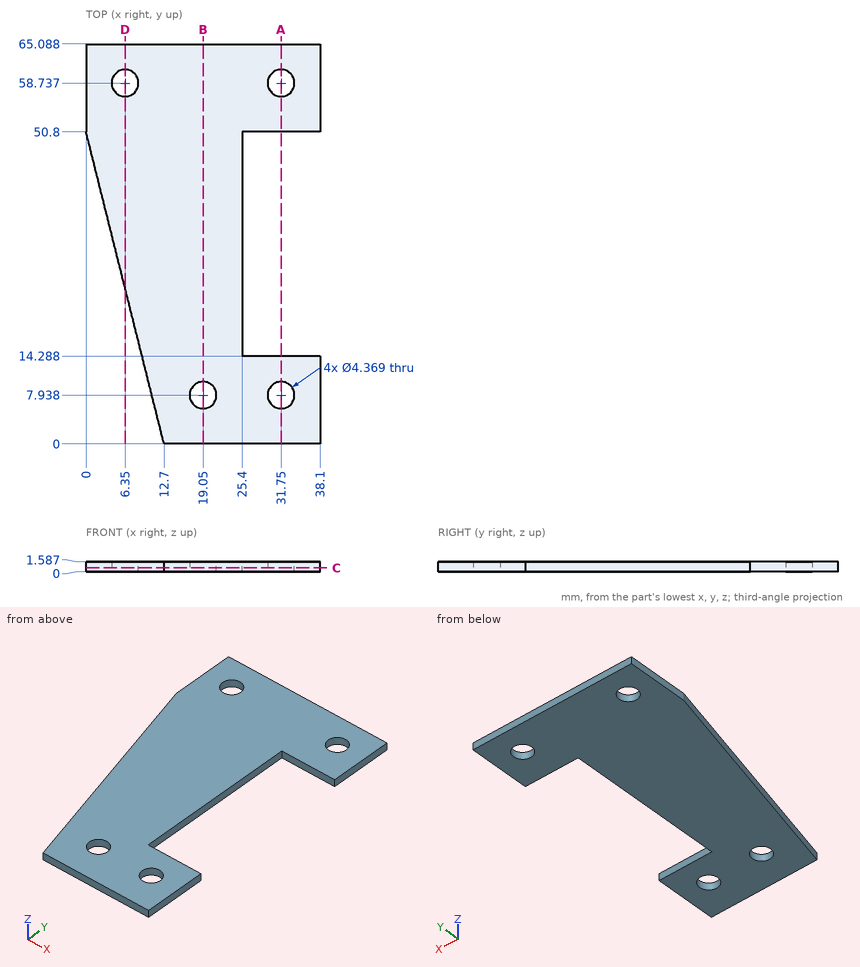
Could you check a few things on this drawing? It's one solid part, dimensions in mm from its lowest x, y, z. Coordinates: 2 decimals unless noted, no trailing zeros. Order: outer loops, then holes, each group sorted by start corner. A loop starts at its lowest first (then second) coordinate and runs counter-clockwise, first axis right, second up.
1) Imagine slicing it at A-A on x = 31.75. List the corners of the cut face in (y, z) for me.
2) Imagine slicing it at B-B on x = 19.05. List the corners of the cut face in (y, z) for me.
3) I need wall thicknesses on line 1 (Y direction, x = 31.75, z = 0.7); line 2 (Y direction, x = 28, z = 0.4); line 3 (Y direction, x = 20, z = 0.4) (1 decimal). Which ranges of each line are inside material? Lowest first, please.
4) Will this pin go through, and if not, where does the flat tip stop? pin 1 (0.5 mm diameter, centred on y = 34, z = 0.5, fed in from +X).
5) Imagine slicing it at D-D on x = 6.35. List the corners of the cut face in (y, z) for me.
6) Imagine slicing it at C-C on z = 0.6. State how many separate pieces and enclosed holes the cut face has, and give its area (3 significant figures).
Response values:
1. outline: (0, 0) - (5.75, 0) - (5.75, 1.59) - (0, 1.59) - close; (10.12, 0) - (14.29, 0) - (14.29, 1.59) - (10.12, 1.59) - close; (50.8, 0) - (56.55, 0) - (56.55, 1.59) - (50.8, 1.59) - close; (60.92, 0) - (65.09, 0) - (65.09, 1.59) - (60.92, 1.59) - close
2. outline: (0, 0) - (5.75, 0) - (5.75, 1.59) - (0, 1.59) - close; (10.12, 0) - (65.09, 0) - (65.09, 1.59) - (10.12, 1.59) - close
3. line 1: y = 0 to 5.75, 10.12 to 14.29, 50.8 to 56.55, 60.92 to 65.09
3. line 2: y = 0 to 14.29, 50.8 to 65.09
3. line 3: y = 0 to 6, 9.9 to 65.1
4. pin 1: stops at x = 25.4
5. outline: (25.4, 0) - (56.55, 0) - (56.55, 1.59) - (25.4, 1.59) - close; (60.92, 0) - (65.09, 0) - (65.09, 1.59) - (60.92, 1.59) - close
6. separate pieces: 1
6. enclosed holes: 4
6. area: 1,630 mm2
